from build123d import *

# Parameters (mm, degrees)
F1_DEPTH = 3.5
F2_R     = 11.25
F3_DEPTH = 3.501
F4_R     = 1


with BuildPart() as f1:
    # F0 (on Top) → F1 (new body)
    with BuildSketch(Plane.XY):
        with BuildLine():
            ThreePointArc((-2.415318, -12.26443), (7.939097, -9.655089), (12.5, 0))
            ThreePointArc((12.5, 0), (-6.292003, 10.800958), (-6.165711, -10.873546))
            ThreePointArc((-6.165711, -10.873546), (-4.346511, -11.719976), (-2.415318, -12.26443))
        make_face()
        with BuildLine():
            ThreePointArc((-2.415318, -12.26443), (-4.346511, -11.719976), (-6.165711, -10.873546))
            Line((-6.165711, -10.873546), (-11.688228, -25.764521))
            Line((-11.688228, -25.764521), (-7.937836, -27.155404))
            Line((-7.937836, -27.155404), (-2.415318, -12.26443))
        make_face()
    extrude(amount=F1_DEPTH)

    # F2 (on face) → F3 (cut, through all)
    with BuildSketch(Plane(origin=(0, 0, 0), x_dir=(1, 0, 0), z_dir=(0, 0, -1))):
        Circle(F2_R)
    extrude(amount=-F3_DEPTH, mode=Mode.SUBTRACT)

    # F4
    f4_edges = [f1.edges().sort_by_distance(p)[0] for p in [
        (-7.937836, -27.155404, 1.75),
        (-11.688228, -25.764521, 1.75),
        (-2.415318, -12.26443, 1.75),
        (-6.165711, -10.873546, 1.75),
    ]]
    fillet(f4_edges, radius=F4_R)


solid = f1.part
The listing builds one solid part. Answer for the finished solid, in the listing's coordinates (mm). A direction names the side the tool comes from. Round coordinates to 2 decimals unless told otherwise and drop trailing zeros. Write each loop counter-clockwise with the first axis right and the second up, starting at its lowest first coordinate (ties: lowest second). Pieces come first, ordered by that corner, then holes. Notation, with made-up numbers: M -28.75,69 L -18.75,69 A25 ccw -18.75,94 Z; hole C 88.5,-24.5 d3. An arc over 180 degrees is marked long. Write each question's results on one line, items separated by ' | '. Start each with the question number.
Item 1: The mould has two halves that part along X. Classify faces 1 (the cylindrical face through (-6.44, -10.98, 1.77)), 2 (the flat face through (-5.18, -19.72, 1.73)), 3 (the cylindrical face through (-2.27, -12.52, 1.77)): +X half, -X half, draft (parallel to the pull), parting line (faces both ways), or undercut.
Item 2: Find section B-B on y = 7.5. Write down the section's boundary in (x, z), and give its area (3 significant figures).
Item 3: Which of the six approach directions +Z, -Z, +X, -X, +Y, -Y give full straight-line access (tool end or side, diameter ignored) to faces 4 (the flat face through (-8.86, -18.14, 1.73)), 5 (the flat face through (-6, -10, 0))?
Item 4: Find section A-A on x = 0. Write down the section's boundary in (y, z).
Item 5: Find section C-C on z = 1.15. Write down the section's boundary in (x, y), and give its area (3 significant figures).
Item 6: Given pin 1 Ø2 at (x, z) = (-3.5, 2) entering from +Y; pin 2 Ø1.5 at (y, z) = (-8.5, 2.5) entering from +X, each flat-ended and moving along its own axis, determine where each tip first touches the part or whether it passes through.
Item 7: Straight lines are drawn through the part: probe 1 along Y at (x, z) = (0, 1.3); probe 2 along X at (y, z) = (-6.5, 0.2); probe 3 along Y at (x, z) = (10.25, 2.6). For each, find the intervals that lie inside material, in ascending order.
Answer block:
1) face 1: -X half | face 2: +X half | face 3: undercut
2) outline: M -10,0 L -8.39,0 L -8.39,3.5 L -10,3.5 Z; M 8.39,0 L 10,0 L 10,3.5 L 8.39,3.5 Z | area: 11.3 mm²
3) face 4: +Z, -Z, -X | face 5: -Z, +X, -X, +Y, -Y
4) outline: M -12.5,0 L -11.25,0 L -11.25,3.5 L -12.5,3.5 Z; M 11.25,0 L 12.5,0 L 12.5,3.5 L 11.25,3.5 Z
5) outline: M -11.34,-24.83 A1 ccw -10.75,-26.11 L -8.88,-26.81 A1 ccw -7.59,-26.22 L -2.7,-13.04 A1 cw -1.63,-12.39 A12.5 ccw long -6.84,-10.46 A1 cw -6.45,-11.65 Z; hole C 0,0 d22.5 | area: 156 mm²
6) pin 1: stops at y = 12.25 | pin 2: stops at x = 9.81
7) probe 1: y = -12.5 to -11.25, 11.25 to 12.5 | probe 2: x = -10.68 to -9.18, 9.18 to 10.68 | probe 3: y = -7.15 to -4.64, 4.64 to 7.15
